Geometry check sheet. Reference: the model listing, model coordinates, mm. Face numbers are marked on the shaded views. Round coordinates to 2 decimals unless told otherwise and drop trailing zeros. Order: outer loops, then holes, each group sorted by start corner. A loop starts at its lowest first (then second) coordinate and runs counter-clockwise, first axis right, second up.
(1) Material ranges on line 1 along Y through (x, z) = (-25, 4); line 2 along X through (y, z) = (2.75, 5.75); line 3 along X through (y, z) = (-9.25, 4.25), recorded low to high.
(2) Release check for a two-part mould opening along Y. For the marked faces 1, 2, 3 and 4 record: +Y half, -Y half, draft (parallel to the pull), parting line (faces both ways), or undercut.
(3) Sectioned sample at C-C (z = 3.75). Give the number of separate pieces and of enclosed holes in the cut face, plus the area to 3 significant figures.
(4) Sectioned sample at D-D (x = -19.5). Record the boundary of the cut face in (y, z), plus the area to 3 significant figures.
(5) Sectioned sample at B-B (y = 0). Record the boundary of the cut face in (x, z).
(6) Go/stop test with flat-tipped pins: pin 1 (2 mm diameter, centred on x = -9, z = 2.5, fed in from -Y); pin 2 (3 mm diameter, centred on x = 27.5, z = 3.5, fed in from -Y). Record where each tip stops, or that it passes through.
(7) Sectioned sample at A-A (x = 0). Record the boundary of the cut face in (y, z).
from build123d import *

# Parameters (mm, degrees)
F0_R     = 11
F1_DEPTH = 6.95
F2_R     = 5


with BuildPart() as f1:
    # F0 (on Top) → F1 (new body)
    with BuildSketch(Plane.XY):
        with BuildLine():
            ThreePointArc((12.5, -5.09902), (38.5, 0), (12.5, 5.09902))
            ThreePointArc((12.5, 5.09902), (0, 13.5), (-12.5, 5.09902))
            ThreePointArc((-12.5, 5.09902), (-38.5, 0), (-12.5, -5.09902))
            ThreePointArc((-12.5, -5.09902), (0, -13.5), (12.5, -5.09902))
        make_face()
        with Locations((-25, 0)):
            Circle(F0_R, mode=Mode.SUBTRACT)
        Circle(F0_R, mode=Mode.SUBTRACT)
        with Locations((25, 0)):
            Circle(F0_R, mode=Mode.SUBTRACT)
    extrude(amount=F1_DEPTH)

    # F2
    f2_edges = [f1.edges().sort_by_distance(p)[0] for p in [
        (-12.5, -5.09902, 3.475),
        (12.5, -5.09902, 3.475),
        (12.5, 5.09902, 3.475),
        (-12.5, 5.09902, 3.475),
    ]]
    fillet(f2_edges, radius=F2_R)


solid = f1.part
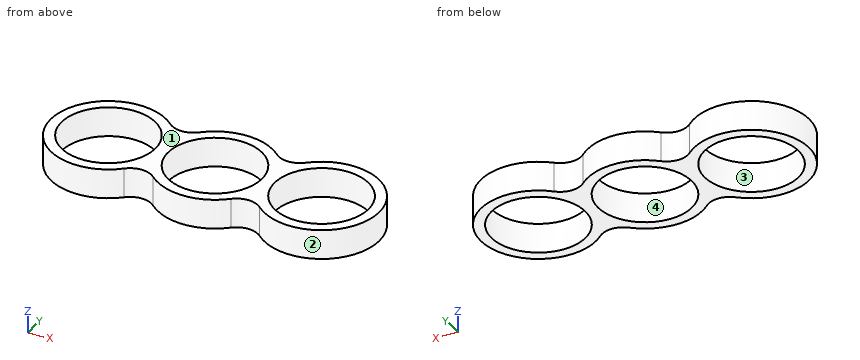
Answer below:
1. line 1: y = -13.5 to -11, 11 to 13.5
1. line 2: x = -38.22 to -35.65, -14.35 to -10.65, 10.65 to 14.35, 35.65 to 38.22
1. line 3: x = -34.83 to -30.95, -19.05 to -14.9, -10.1 to -5.95, 5.95 to 10.1, 14.9 to 19.05, 30.95 to 34.83
2. face 1: draft
2. face 2: parting line
2. face 3: undercut
2. face 4: undercut
3. separate pieces: 1
3. enclosed holes: 3
3. area: 581 mm2
4. outline: (-12.33, 0) - (-9.53, 0) - (-9.53, 6.95) - (-12.33, 6.95) - close; (9.53, 0) - (12.33, 0) - (12.33, 6.95) - (9.53, 6.95) - close
4. area: 39.0 mm2
5. outline: (-38.5, 0) - (-36, 0) - (-36, 6.95) - (-38.5, 6.95) - close; (-14, 0) - (-11, 0) - (-11, 6.95) - (-14, 6.95) - close; (11, 0) - (14, 0) - (14, 6.95) - (11, 6.95) - close; (36, 0) - (38.5, 0) - (38.5, 6.95) - (36, 6.95) - close
6. pin 1: stops at y = -10.87
6. pin 2: stops at y = -13.46
7. outline: (-13.5, 0) - (-11, 0) - (-11, 6.95) - (-13.5, 6.95) - close; (11, 0) - (13.5, 0) - (13.5, 6.95) - (11, 6.95) - close
